Here's how the part is built. I have some questions about the finished solid (model axes, mm). Face numbers are marked on the shaded views. A direction names the side the tool comes from. Round coordinates to 2 decimals unless told otherwise and drop trailing zeros. Loops run counter-clockwise (first coordinate to the right, second up) from the corner with the lowest first, then second, coordinate; pieces in that order, holes last. Notation, with made-up numbers: M -33.5,-4.75 L 14.5,-4.75 A16 cw 14.5,16.25 Z; hole C 41.5,15 d8. An arc over 180 degrees is marked long. Use a Markdown table: item, result.
from build123d import *

# Parameters (mm, degrees)
SKETCH1_R           = 22.5
BOSS_EXTRUDE1_DEPTH = 10
SKETCH2_R           = 30
BOSS_EXTRUDE2_DEPTH = 20
SKETCH3_R           = 16.5
CUT_EXTRUDE2_DEPTH  = 5


with BuildPart() as part:
    # Sketch1 → Boss-Extrude1 (new body)
    with BuildSketch(Plane(origin=(0, 0, 0), x_dir=(1, 0, 0), z_dir=(0, 1, 0))):
        Circle(SKETCH1_R)
    extrude(amount=BOSS_EXTRUDE1_DEPTH)

    # Sketch2 → Boss-Extrude2 (add)
    with BuildSketch(Plane(origin=(0, 10, 0), x_dir=(1, 0, 0), z_dir=(0, 1, 0))):
        Circle(SKETCH2_R)
    extrude(amount=BOSS_EXTRUDE2_DEPTH)

    # Sketch3 → Cut-Extrude2 (cut)
    with BuildSketch(Plane.XZ):
        with BuildLine():
            ThreePointArc((-14.551420086, 2.778571429), (0, 11.5), (14.551420086, 2.778571429))
            Line((14.551420086, 2.778571429), (4.83856504, 20.948467447))
            ThreePointArc((4.83856504, 20.948467447), (0, 21.5), (-4.83856504, 20.948467447))
            Line((-4.83856504, 20.948467447), (-14.551420086, 2.778571429))
        make_face()
        with Locations((0, -5)):
            Circle(SKETCH3_R)
    extrude(amount=-CUT_EXTRUDE2_DEPTH, mode=Mode.SUBTRACT)


solid = part.part
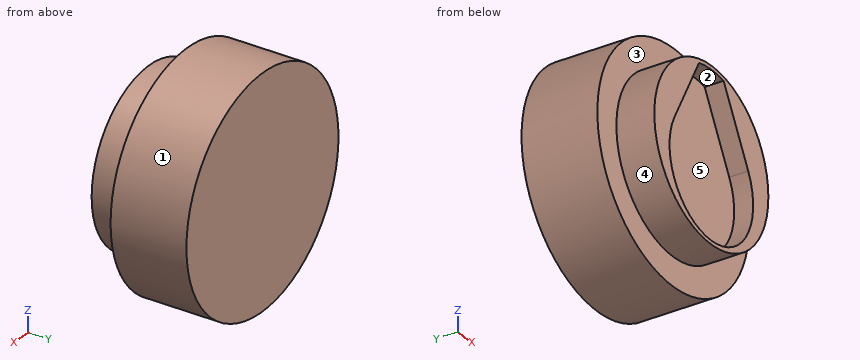
1. Imagine slicing it at C-C, the plane y = 15.5. Write out the boundary of the cut face in (x, z).
Answer sheet:
| item | result |
|---|---|
| outline | C 0,0 d60 |
2. Imagine slicing it at D-D, the plane x = 20. Write out the boundary of the cut face in (y, z).
Answer sheet:
| item | result |
|---|---|
| outline | M 0,-10.31 L 10,-10.31 L 10,-22.36 L 30,-22.36 L 30,22.36 L 10,22.36 L 10,10.31 L 0,10.31 Z |
3. Imagine slicing it at B-B, the plane z = 0. Write out the boundary of the cut face in (x, y), then the cut area to 3 significant figures.
Answer sheet:
| item | result |
|---|---|
| outline | M -30,10 L -22.5,10 L -22.5,0 L -15.72,0 L -15.72,5 L 15.72,5 L 15.72,0 L 22.5,0 L 22.5,10 L 30,10 L 30,30 L -30,30 Z |
| area | 1,490 mm2 |
4. I need wall thicknesses on probe 1 along Y at (x, z) = (6, 15.5); probe 2 along Y at (x, z) = (23, 4); probe 3 along X at (y, z) = (4.25, -19.5). Which ranges of each line are inside material? Lowest first, please. Write a range as from..to.
Answer sheet:
| item | result |
|---|---|
| probe 1 | 5..30 |
| probe 2 | 10..30 |
| probe 3 | -11.22..-7.87, 7.87..11.22 |
5. Which directions (+Z, -Z, +X, -X, +Y, -Y) give clear straight access to the entire face, cutting with the end or side of a thin tool? Please do the marked faces 1 and 2.
Answer sheet:
| item | result |
|---|---|
| face 1 | +Y, -Y |
| face 2 | -Y |
6. Imagine slicing it at A-A, the plane x = 0. Write out the boundary of the cut face in (y, z), then the cut area to 4 significant figures.
Answer sheet:
| item | result |
|---|---|
| outline | M 0,-22.5 L 10,-22.5 L 10,-30 L 30,-30 L 30,30 L 10,30 L 10,22.5 L 0,22.5 L 0,21.5 L 5,21.5 L 5,-21.5 L 0,-21.5 Z |
| area | 1,435 mm2 |
7. We'd pull the mould along Z, two halves only. Please class the marked faces 3, 4 and 5: +Z half, -Z half, draft (parallel to the pull), parting line (faces both ways), or undercut.
Answer sheet:
| item | result |
|---|---|
| face 3 | draft |
| face 4 | parting line |
| face 5 | undercut |
8. For pin 1 Ø4 at (y, z) = (5.5, 10) entering from +X; pin 2 Ø5 at (y, z) = (5.5, -14) entering from +X; pin 3 Ø16.5 at (x, z) = (5, -4) entering from -Y, each with a flat end and sliding along its axis, tell me the tip position at first contact or that it passes through.
Answer sheet:
| item | result |
|---|---|
| pin 1 | x = 21.03 |
| pin 2 | x = 19.34 |
| pin 3 | y = 5 |
